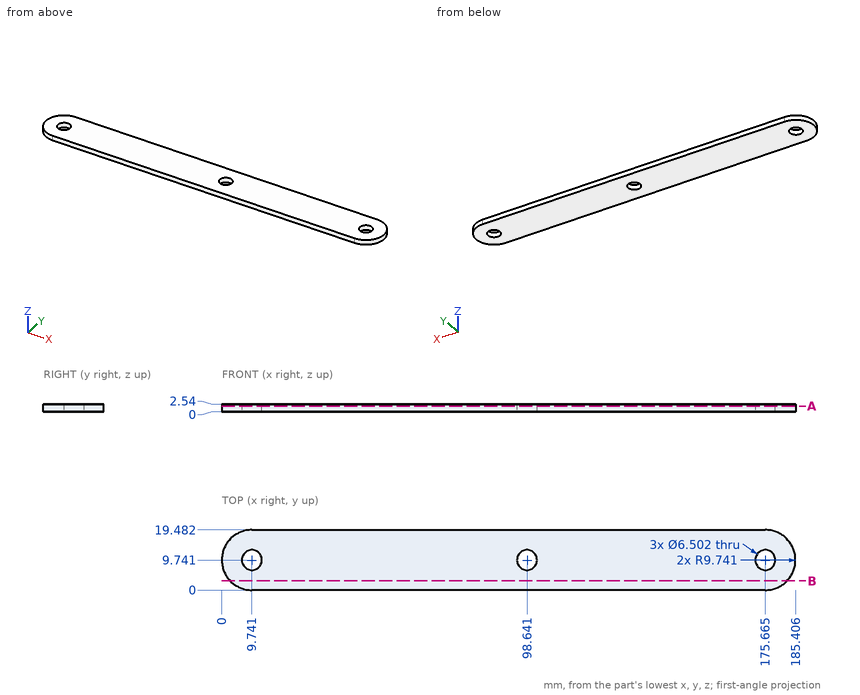
The drawing under review shows one solid part. Ordinate dimensions are in mm from its lowest x, y, z. Give positions to 0.01 mm unless a question says otherwise; leave off trailing zeros. Loops run counter-clockwise (first coordinate to the right, second up) from the corner with the lowest first, then second, coordinate; pieces in that order, holes last. Notation, with made-up numbers: M 24,21 L 49,21 A18 cw 49,37 Z; hole C 38,68.5 d9. An arc over 180 degrees is marked long. One line per item, written item: value. Start each with the question number.
Q1. Add section A-A (z = 1.85). Give the boundary of the cut face in (x, y) (1 decimal).
Q2. For L1, parallel to X at y = 10.25, z = 0.25 (1 decimal); L2, parallel to X at y = 7.75, z = 1.75 (1 decimal); L3, parallel to X at y = 1.75, z = 1.45 (1 decimal), list the stretches that pass through material, from the lowest coordinate up.
Q3. Add section B-B (y = 3). Give the boundary of the cut face in (x, z), and give its area (3 significant figures).
Q4. Clearance check with a flat-ended pin moving along its axis: pin 1 Ø1 at (y, z) = (9, 2) entering from -X. State where the tip first meets the part, or that it passes through.
Reply:
1. outline: M 9.7,0 L 175.7,0 A9.7 ccw 175.7,19.5 L 9.7,19.5 A9.7 ccw Z; hole C 9.7,9.7 d6.5; hole C 98.6,9.7 d6.5; hole C 175.7,9.7 d6.5
2. L1: 0 to 6.5, 13 to 95.4, 101.9 to 172.5, 178.9 to 185.4
2. L2: 0.2 to 7.2, 12.3 to 96.1, 101.2 to 173.1, 178.2 to 185.2
2. L3: 4.2 to 181.2
3. outline: M 2.71,0 L 182.7,0 L 182.7,2.54 L 2.71,2.54 Z
3. area: 457 mm²
4. pin 1: x = 0
